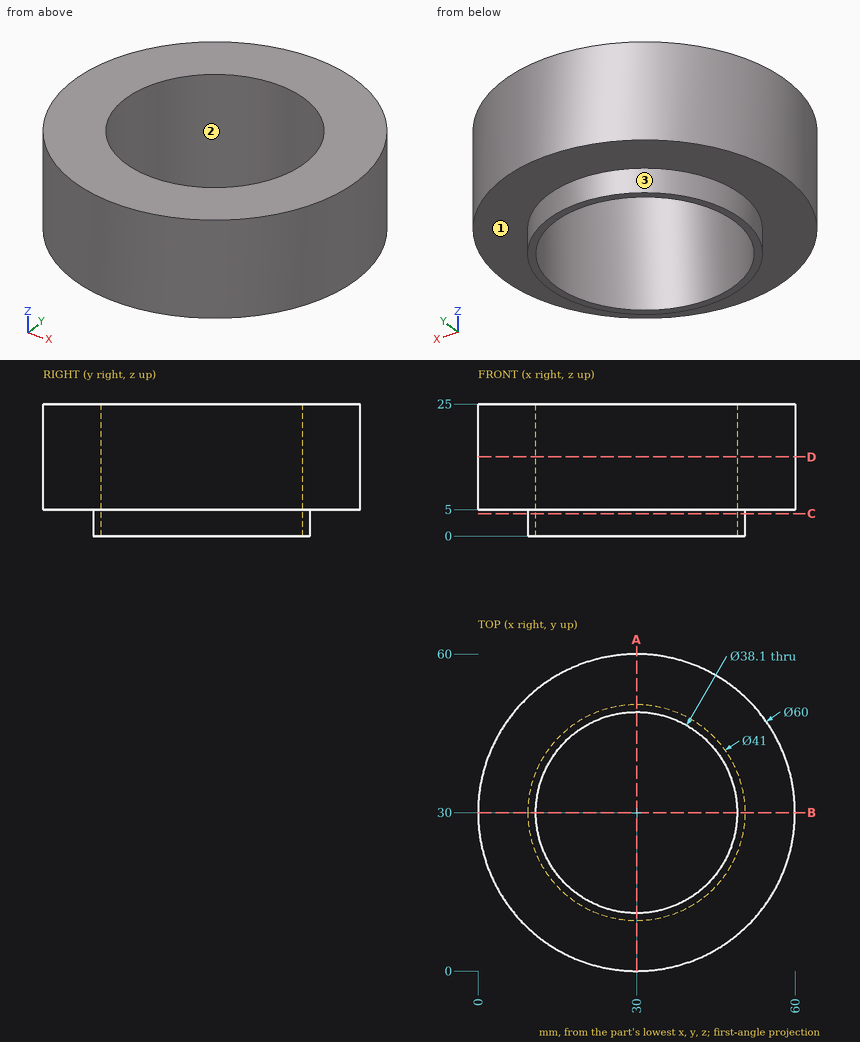
The figure shows three views and two pictorial views of one solid part (mm, origin at its lowest corner). Answer the questions. Give positions to 0.01 mm unless a question says otherwise; leave off trailing zeros. Write each loop counter-clockwise with the first axis right and the second up, starting at its lowest first coordinate (ties: lowest second). Pieces come first, ordered by that corner, then holes. Notation, with made-up numbers: (76.5, -20) - (113.5, -20) arc R10 cw to (113.5, -5) - close; hole circle Ø2 at (17, 15). An arc over 180 degrees is marked (long way). Return JSON: item names as keys, results as strings.
Q1. Consider line 1 along Y through (x, z) = (30, 7.5); line 2 along X through (y, z) = (39, 13.25); line 3 along X through (y, z) = (36, 22.75). Determine where each line is inside the solid, lowest interval first. Write a range as [from, to].
Reply:
{"line 1": "[0, 10.95], [49.05, 60]", "line 2": "[1.38, 13.21], [46.79, 58.62]", "line 3": "[0.61, 11.92], [48.08, 59.39]"}
Q2. A cutting plane is placed at C-C, the plane z = 4.25. Determine the outline of the cut face in (x, y), and give its area (3 significant figures).
Reply:
{"outline": "circle Ø41 at (30, 30); hole circle Ø38.1 at (30, 30)", "area": "180 mm²"}
Q3. A cutting plane is placed at A-A, the plane x = 30. Determine the outline of the cut face in (y, z), and give its area (4 significant figures).
Reply:
{"outline": "(0, 5) - (9.5, 5) - (9.5, 0) - (10.95, 0) - (10.95, 25) - (0, 25) - close; (49.05, 0) - (50.5, 0) - (50.5, 5) - (60, 5) - (60, 25) - (49.05, 25) - close", "area": "452.5 mm²"}
Q4. For a pull along Y with two mould halves and no side action, classify the marked faces 1, 2 and 3 as released by +Y, released by -Y, zero draft, split by the parting line, or undercut.
Reply:
{"face 1": "zero draft", "face 2": "undercut", "face 3": "split by the parting line"}
Q5. A cutting plane is placed at D-D, the plane z = 15. Determine the outline of the cut face in (x, y).
Reply:
{"outline": "circle Ø60 at (30, 30); hole circle Ø38.1 at (30, 30)"}
Q6. Given P1, Ø6, axis at x = 40, z = 13.5, coming from the +Y side; P2, Ø2, axis at x = 24, z = 19.5, coming from the -Y side; P3, Ø1.5, axis at y = 34, z = 8.5, coming from the -X side, each flat-ended and moving along its own axis, determine where each tip first touches the part or whether it passes through.
Reply:
{"P1": "y = 59.17", "P2": "y = 0.42", "P3": "x = 0.18"}
